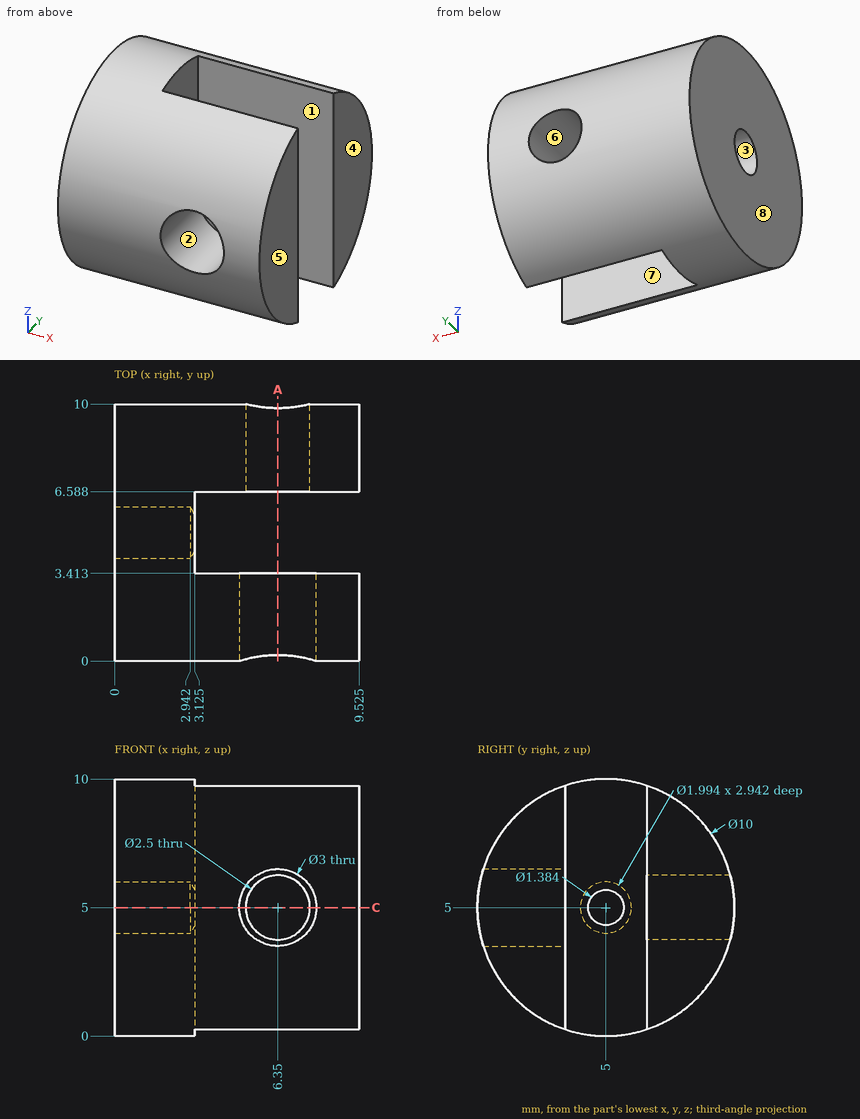
Here's the drawing with two shaded views (mm, measured from the low corner). I have some questions. A direction names the side the tool comes from. Coordinates: 2 decimals unless noted, no trailing zeros. Write each loop counter-clockwise with the first axis right and the second up, starting at its lowest first coordinate (ties: lowest second). Pieces come first, ordered by that corner, then holes. Notation, with made-up numbers: (-9.75, -21) -> (1.25, -21) arc R24 ccw to (1.25, 0) -> close; hole circle Ø6 at (88.5, -20.75). An arc over 180 degrees is marked (long way). Use a Markdown table: item, result. Add a question column.
(1) I'm going to push flat-ended pins straight in: P1, Ø5, axis at x = 7.5, z = 8.5, coming from the +Y side; P2, Ø2.5, axis at y = 5, z = 7, coming from the +X side (1 decimal); P3, Ø1.5, axis at x = 3, y = 6.5, coming from the +Z side; P4, Ø2, axis at x = 6.35, z = 5, coming from the +Y side. Where does each tip first touch, or does it pass through?
(2) Please list where these lines run through material, in increasing order: line 1 (Z direction, x = 1.15, y = 5); line 2 (X direction, y = 3.25, z = 6) (1 decimal); line 3 (Y direction, x = 5.25, z = 8) (1 decimal).
(3) If we section it at C-C, the plane z = 5: State how many separate pieces and enclosed holes the cut face has.
(4) We'd pull the mould along X, two halves only. Please class the marked faces 5, 6, 7 and 8: +X half, -X half, draft (parallel to the pull), parting line (faces both ways), or undercut.
(5) If we section it at A-A, the plane x = 6.35: Write out the boundary of the cut face in (y, z).
(6) For the marked faces 1, 2, 3 and 4, which set-ups out of +Z, -Z, +X, -X, +Y, -Y let a thin tool reach every point of the face, with its end or its side?
Outcome:
| question | item | result |
|---|---|---|
| 1 | P1 | stops at y = 9.9 |
| 1 | P2 | stops at x = 3.1 |
| 1 | P3 | stops at z = 9.94 |
| 1 | P4 | passes through |
| 2 | line 1 | z = 0 to 4, 6 to 10 |
| 2 | line 2 | x = 0 to 5.2, 7.5 to 9.5 |
| 2 | line 3 | y = 1 to 3.4, 6.6 to 9 |
| 3 | separate pieces | 4 |
| 3 | enclosed holes | 0 |
| 4 | face 5 | +X half |
| 4 | face 6 | undercut |
| 4 | face 7 | draft |
| 4 | face 8 | -X half |
| 5 | outline | (0.23, 3.5) arc R5 ccw to (3.41, 0.26) -> (3.41, 3.5) -> close; (0.23, 6.5) -> (3.41, 6.5) -> (3.41, 9.74) arc R5 ccw to start; (6.59, 0.26) arc R5 ccw to (9.84, 3.75) -> (6.59, 3.75) -> close; (6.59, 6.25) -> (9.84, 6.25) arc R5 ccw to (6.59, 9.74) -> close |
| 6 | face 1 | +Z, -Z, +X |
| 6 | face 2 | -Y |
| 6 | face 3 | -X |
| 6 | face 4 | +Z, -Z, +X, +Y, -Y |
